```python
from build123d import *

# Parameters (mm, degrees)
BOSS_EXTRUDE1_DEPTH             = 600
BOSS_EXTRUDE2_DEPTH             = 10
FILLET1_R                       = 10
FILLET1_OF_MIRROR2_R            = 10
BOSS_EXTRUDE3_REACH             = 718.356
SKETCH3_W                       = 200
SKETCH3_H                       = 25
BOSS_EXTRUDE3_DIRECTION_2_DEPTH = 220
SKETCH4_W                       = 200
SKETCH4_H                       = 96.738577366
BOSS_EXTRUDE4_DEPTH             = 5
FILLET3_R                       = 10
SKETCH5_R                       = 5
CUT_EXTRUDE1_DEPTH              = 5
CUT_EXTRUDE3_REACH              = 731.903
CUT_EXTRUDE3_DIRECTION_2_REACH  = 731.903


with BuildPart() as part:
    # Sketch1 → Boss-Extrude1 (new, symmetric)
    with BuildSketch(Plane.XY):
        with BuildLine():
            Line((301.229416671, 150), (303.350737014, 147.878679656))
            ThreePointArc((303.350737014, 147.878679656), (175.223022732, 43.605710521), (15.886569686, 0))
            ThreePointArc((15.886569686, 0), (0.006557212, 14.530298176), (15, 29.973776885))
            ThreePointArc((15, 29.973776885), (170.230890365, 61.093138188), (301.229416671, 150))
        make_face()
    extrude(amount=BOSS_EXTRUDE1_DEPTH, both=True)

    # Sketch2 → Boss-Extrude2 (add)
    with BuildSketch(Plane.XY.offset(600)):
        Polygon((-47.601621627, 79.452155227), (-47.601621627, -15.547844773), (60.841138561, -61.045034952), (323.670396802, 61.514260953), (331.950192363, 156.152757271), (319.450192363, 177.803392366), align=None)
    boss_extrude2 = extrude(amount=BOSS_EXTRUDE2_DEPTH)

    # Fillet1
    fillet1_edges = [part.edges().sort_by_distance(p)[0] for p in [
        (319.450192363, 177.803392366, 605),
        (-47.601621627, 79.452155227, 605),
        (-47.601621627, -15.547844773, 605),
        (60.841138561, -61.045034952, 605),
        (323.670396802, 61.514260953, 605),
        (331.950192363, 156.152757271, 605),
    ]]
    fillet(fillet1_edges, radius=FILLET1_R)

    # Mirror2: Boss-Extrude2 across plane
    add(boss_extrude2.mirror(Plane.XY))

    # Fillet1 of Mirror2
    fillet1_of_mirror2_edges = [part.edges().sort_by_distance(p)[0] for p in [
        (319.450192363, 177.803392366, -605),
        (-47.601621627, 79.452155227, -605),
        (-47.601621627, -15.547844773, -605),
        (60.841138561, -61.045034952, -605),
        (323.670396802, 61.514260953, -605),
        (331.950192363, 156.152757271, -605),
    ]]
    fillet(fillet1_of_mirror2_edges, radius=FILLET1_OF_MIRROR2_R)

    # Sketch3 → Boss-Extrude3 (add, up to next)
    with BuildSketch(Plane(origin=(0, 0, 0), x_dir=(1, 0, 0), z_dir=(0, 1, 0)), mode=Mode.PRIVATE) as boss_extrude3_sk1:
        with Locations((158.114708335, -262.5)):
            Rectangle(SKETCH3_W, SKETCH3_H)
    boss_extrude3_tool1 = extrude(boss_extrude3_sk1.sketch, amount=BOSS_EXTRUDE3_REACH, mode=Mode.PRIVATE) - part.part
    boss_extrude3 = boss_extrude3_tool1.solids().sort_by_distance((158.114708, 0, 262.5))[0]
    add(boss_extrude3)

    # Sketch3 → Boss-Extrude3 direction 2 (add)
    with BuildSketch(Plane(origin=(0, 0, 0), x_dir=(1, 0, 0), z_dir=(0, 1, 0))):
        with Locations((158.114708335, -262.5)):
            Rectangle(SKETCH3_W, SKETCH3_H)
    boss_extrude3_direction_2 = extrude(amount=-BOSS_EXTRUDE3_DIRECTION_2_DEPTH)

    # Mirror3: Boss-Extrude3, Boss-Extrude3 direction 2 across plane
    add(boss_extrude3.mirror(Plane.XY))
    add(boss_extrude3_direction_2.mirror(Plane.XY))

    # Sketch4 → Boss-Extrude4 (add)
    with BuildSketch(Plane.XZ.offset(220)):
        with Locations((158.114708335, 262.5)):
            Rectangle(SKETCH4_W, SKETCH4_H)
    boss_extrude4 = extrude(amount=BOSS_EXTRUDE4_DEPTH)

    # Mirror6: Boss-Extrude4 across plane
    add(boss_extrude4.mirror(Plane.XY))

    # Fillet3
    fillet3_edges = [part.edges().sort_by_distance(p)[0] for p in [
        (158.114708335, -220, 275),
        (158.114708335, -220, 250),
        (158.114708335, -220, -250),
        (158.114708335, -220, -275),
    ]]
    fillet(fillet3_edges, radius=FILLET3_R)

    # Sketch5 → Cut-Extrude1 (cut)
    with BuildSketch(Plane.XZ.offset(225)):
        with Locations(Location((83.114708335, 295.869288683, 0), (0, 0, 270))):
            Circle(SKETCH5_R)
        with Locations(Location((184.214708335, 295.869288683, 0), (0, 0, 270))):
            Circle(SKETCH5_R)
        with Locations(Location((184.214708335, 229.130711317, 0), (0, 0, 270))):
            Circle(SKETCH5_R)
        with Locations(Location((83.114708335, 229.130711317, 0), (0, 0, 270))):
            Circle(SKETCH5_R)
    cut_extrude1 = extrude(amount=-CUT_EXTRUDE1_DEPTH, mode=Mode.SUBTRACT)

    # Mirror7: Cut-Extrude1 across plane
    add(cut_extrude1.mirror(Plane.XY), mode=Mode.SUBTRACT)

    # Sketch8 → Cut-Extrude3 (cut, up to next)
    with BuildSketch(Plane.XY, mode=Mode.PRIVATE) as cut_extrude3_sk1:
        Polygon((258.114708335, 100), (209.210600029, -225), (258.114708335, -225), align=None)
    cut_extrude3_tool1 = extrude(cut_extrude3_sk1.sketch, amount=-CUT_EXTRUDE3_REACH, mode=Mode.PRIVATE) & part.part
    # Sketch8 → Cut-Extrude3 (cut, up to next)
    with BuildSketch(Plane.XY, mode=Mode.PRIVATE) as cut_extrude3_sk2:
        Polygon((192.672505063, -200), (234.626697196, 78.813230948), (77.908149081, -200), align=None)
    cut_extrude3_tool2 = extrude(cut_extrude3_sk2.sketch, amount=-CUT_EXTRUDE3_REACH, mode=Mode.PRIVATE) & part.part
    # Sketch8 → Cut-Extrude3 (cut, up to next)
    with BuildSketch(Plane.XY, mode=Mode.PRIVATE) as cut_extrude3_sk3:
        Polygon((77.406994689, -169.918867637), (203.697901707, 54.761466943), (77.406994689, -7.882832173), align=None)
    cut_extrude3_tool3 = extrude(cut_extrude3_sk3.sketch, amount=-CUT_EXTRUDE3_REACH, mode=Mode.PRIVATE) & part.part
    add(cut_extrude3_tool1.solids().sort_by_distance((241.813339, -116.666667, 0))[0], mode=Mode.SUBTRACT)
    add(cut_extrude3_tool2.solids().sort_by_distance((168.40245, -107.062256, 0))[0], mode=Mode.SUBTRACT)
    add(cut_extrude3_tool3.solids().sort_by_distance((119.503964, -41.013411, 0))[0], mode=Mode.SUBTRACT)

    # Sketch8 → Cut-Extrude3 direction 2 (cut, up to next)
    with BuildSketch(Plane.XY, mode=Mode.PRIVATE) as cut_extrude3_direction_2_sk1:
        Polygon((258.114708335, 100), (209.210600029, -225), (258.114708335, -225), align=None)
    cut_extrude3_direction_2_tool1 = extrude(cut_extrude3_direction_2_sk1.sketch, amount=CUT_EXTRUDE3_DIRECTION_2_REACH, mode=Mode.PRIVATE) & part.part
    # Sketch8 → Cut-Extrude3 direction 2 (cut, up to next)
    with BuildSketch(Plane.XY, mode=Mode.PRIVATE) as cut_extrude3_direction_2_sk2:
        Polygon((192.672505063, -200), (234.626697196, 78.813230948), (77.908149081, -200), align=None)
    cut_extrude3_direction_2_tool2 = extrude(cut_extrude3_direction_2_sk2.sketch, amount=CUT_EXTRUDE3_DIRECTION_2_REACH, mode=Mode.PRIVATE) & part.part
    # Sketch8 → Cut-Extrude3 direction 2 (cut, up to next)
    with BuildSketch(Plane.XY, mode=Mode.PRIVATE) as cut_extrude3_direction_2_sk3:
        Polygon((77.406994689, -169.918867637), (203.697901707, 54.761466943), (77.406994689, -7.882832173), align=None)
    cut_extrude3_direction_2_tool3 = extrude(cut_extrude3_direction_2_sk3.sketch, amount=CUT_EXTRUDE3_DIRECTION_2_REACH, mode=Mode.PRIVATE) & part.part
    add(cut_extrude3_direction_2_tool1.solids().sort_by_distance((241.813339, -116.666667, 0))[0], mode=Mode.SUBTRACT)
    add(cut_extrude3_direction_2_tool2.solids().sort_by_distance((168.40245, -107.062256, 0))[0], mode=Mode.SUBTRACT)
    add(cut_extrude3_direction_2_tool3.solids().sort_by_distance((119.503964, -41.013411, 0))[0], mode=Mode.SUBTRACT)


solid = part.part
```
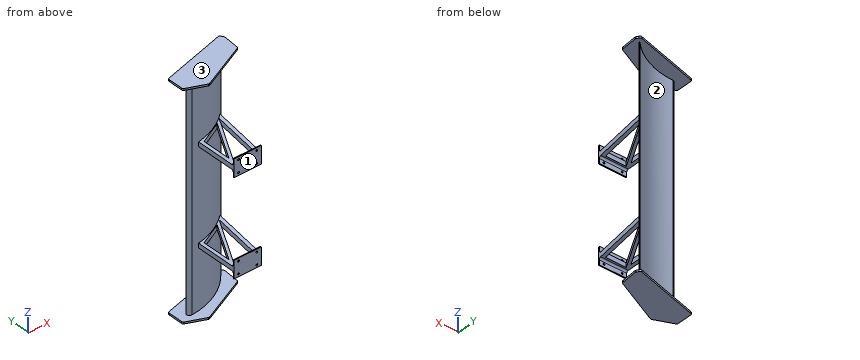
Geometry: final body of the model. Coordinates: model frame, mm. Face numbers are marked on the shaded views. Give positions to 0.01 mm unless a question says otherwise; leave off trailing zeros. Order: outer loops, then holes, each group sorted by start corner. A loop starts at its lowest first (then second) coordinate and runs counter-clockwise, first axis right, second up. Notation, with made-up numbers: (-18.75, 78) -> (35.25, 78) arc R16 cw to (35.25, 109) -> close; hole circle Ø11 at (26.5, 38.5). An arc over 180 degrees is marked (long way). Write each question's results on one line, items separated by ' | '. Start each with the question number.
1) Section A-A (y = -29.5). Count the separate pieces of the cut face and the enclosed holes in it, then the cut area to 3 significant figures.
2) Draft query along Z for the marked faces 1, 2 and 3. Return one class per face: pulls with the +Z half, pulls with the -Z half, needs draft (parallel to the pull), parting line crosses it, or undercut.
3) First-contact query: pin 1 (10 mm diameter, centred on x = 270, z = 363, fed in from -Y); pin 2 (8 mm diameter, centred on x = 184.21, z = -229.13, fed in from +Y); pin 3 (12.5 mm diameter, centred on y = -77, z = 268, fed in from +X). Flat tips, straight axial feed; report the tip coordinate or a pass-through.
4) Section B-B (x = -21). Return loops of the section in (y, z), then the cut area to 3 significant figures.
5) Section C-C (z = -396). Return loops of the section in (x, y).
6) Line query: line 1 (Z direction, x = 244, y = 51); line 2 (Z direction, x = 198, y = 104.5); line 3 (X direction, y = -107, z = 258). Output: solid intervals per line, ascending. Write a range as from..to.
Calculated:
1) separate pieces: 8 | enclosed holes: 0 | area: 5,710 mm2
2) face 1: needs draft | face 2: undercut | face 3: pulls with the +Z half
3) pin 1: y = 106.72 | pin 2: y = 69.16 | pin 3: x = 232.42
4) outline: (-26.71, -610) -> (86.58, -610) -> (86.58, -600) -> (-26.71, -600) -> close; (-26.71, 600) -> (86.58, 600) -> (86.58, 610) -> (-26.71, 610) -> close | area: 2,270 mm2
5) outline: (15, 29.97) arc R15 ccw (long way) to (15.89, 0) arc R400 ccw to (303.35, 147.88) -> (301.23, 150) arc R400 cw to start
6) line 1: -610..-600, -275..-250, 250..275, 600..610 | line 2: -610..-600, 600..610 | line 3: 58.11..77.41, 112.77..130.18, 206.67..226.97
